The model under review builds one solid part; all positions refer to its coordinate system, in mm. A direction names the side the tool comes from. Give positions to 0.01 mm unless a question says otherwise; leave off trailing zeros. Loops run counter-clockwise (first coordinate to the right, second up) from the corner with the lowest first, then second, coordinate; pieces in that order, holes last. Notation, with made-up numbers: (67, 25) - (95, 25) arc R22 cw to (95, 31) - close; hole circle Ø7 at (18, 55.5). An arc over 180 degrees is marked (long way). Return JSON: item names as keys, results as strings. Group by question number.
```python
from build123d import *

# Parameters (mm, degrees)
SKETCH1_RX          = 20
SKETCH1_RY          = 15
BOSS_EXTRUDE1_DEPTH = 6


with BuildPart() as part:
    # Sketch1 → Boss-Extrude1 (new body)
    with BuildSketch(Plane.XY):
        with BuildLine():
            Line((735.278050496, 436.653824982), (737.672420097, 436.653824982))
            Line((737.672420097, 436.653824982), (737.672420097, 437.878226994))
            Line((737.672420097, 437.878226994), (742.24679609, 437.878226994))
            Line((742.24679609, 437.878226994), (742.24679609, 431.116067))
            Line((742.24679609, 431.116067), (747.348599543, 431.116067))
            Line((747.348599543, 431.116067), (747.348599543, 427.736067))
            Line((747.348599543, 427.736067), (742.114877809, 427.736067))
            ThreePointArc((742.114877809, 427.736067), (721.48448246, 433.262998961), (700.85408711, 427.736067))
            Line((700.85408711, 427.736067), (695.865635692, 427.736067))
            Line((695.865635692, 427.736067), (695.865635692, 431.116067))
            Line((695.865635692, 431.116067), (700.917916144, 431.116067))
            Line((700.917916144, 431.116067), (700.917916144, 437.878226994))
            Line((700.917916144, 437.878226994), (705.492292137, 437.878226994))
            Line((705.492292137, 437.878226994), (705.492292137, 436.653824982))
            Line((705.492292137, 436.653824982), (707.886661739, 436.653824982))
            Line((707.886661739, 436.653824982), (707.886661739, 437.878226994))
            Line((707.886661739, 437.878226994), (709.486661739, 437.878226994))
            Line((709.486661739, 437.878226994), (709.486661739, 440.973907006))
            Line((709.486661739, 440.973907006), (707.886661739, 440.973907006))
            Line((707.886661739, 440.973907006), (707.886661739, 442.198309018))
            Line((707.886661739, 442.198309018), (705.492292137, 442.198309018))
            Line((705.492292137, 442.198309018), (705.492292137, 440.973907006))
            Line((705.492292137, 440.973907006), (700.917916144, 440.973907006))
            Line((700.917916144, 440.973907006), (700.917916144, 459.426067))
            Line((700.917916144, 459.426067), (700.917916144, 477.878226994))
            Line((700.917916144, 477.878226994), (705.492292137, 477.878226994))
            Line((705.492292137, 477.878226994), (705.492292137, 476.653824982))
            Line((705.492292137, 476.653824982), (707.886661739, 476.653824982))
            Line((707.886661739, 476.653824982), (707.886661739, 477.878226994))
            Line((707.886661739, 477.878226994), (709.486661739, 477.878226994))
            Line((709.486661739, 477.878226994), (709.486661739, 480.973907006))
            Line((709.486661739, 480.973907006), (707.886661739, 480.973907006))
            Line((707.886661739, 480.973907006), (707.886661739, 482.198309018))
            Line((707.886661739, 482.198309018), (705.492292137, 482.198309018))
            Line((705.492292137, 482.198309018), (705.492292137, 480.973907006))
            Line((705.492292137, 480.973907006), (700.917916144, 480.973907006))
            Line((700.917916144, 480.973907006), (700.917916144, 487.736067))
            Line((700.917916144, 487.736067), (695.865635692, 487.736067))
            Line((695.865635692, 487.736067), (695.865635692, 491.116067))
            Line((695.865635692, 491.116067), (700.85408711, 491.116067))
            ThreePointArc((700.85408711, 491.116067), (721.48448246, 485.589135038), (742.114877809, 491.116067))
            Line((742.114877809, 491.116067), (747.348599543, 491.116067))
            Line((747.348599543, 491.116067), (747.348599543, 487.736067))
            Line((747.348599543, 487.736067), (742.24679609, 487.736067))
            Line((742.24679609, 487.736067), (742.24679609, 480.973907006))
            Line((742.24679609, 480.973907006), (737.672420097, 480.973907006))
            Line((737.672420097, 480.973907006), (737.672420097, 482.198309018))
            Line((737.672420097, 482.198309018), (735.278050496, 482.198309018))
            Line((735.278050496, 482.198309018), (735.278050496, 480.973907006))
            Line((735.278050496, 480.973907006), (733.799948182, 480.973907006))
            Line((733.799948182, 480.973907006), (733.799948182, 477.878226994))
            Line((733.799948182, 477.878226994), (735.278050496, 477.878226994))
            Line((735.278050496, 477.878226994), (735.278050496, 476.653824982))
            Line((735.278050496, 476.653824982), (737.672420097, 476.653824982))
            Line((737.672420097, 476.653824982), (737.672420097, 477.878226994))
            Line((737.672420097, 477.878226994), (742.24679609, 477.878226994))
            Line((742.24679609, 477.878226994), (742.24679609, 459.426067))
            Line((742.24679609, 459.426067), (742.24679609, 440.973907006))
            Line((742.24679609, 440.973907006), (737.672420097, 440.973907006))
            Line((737.672420097, 440.973907006), (737.672420097, 442.198309018))
            Line((737.672420097, 442.198309018), (735.278050496, 442.198309018))
            Line((735.278050496, 442.198309018), (735.278050496, 440.973907006))
            Line((735.278050496, 440.973907006), (733.799948182, 440.973907006))
            Line((733.799948182, 440.973907006), (733.799948182, 437.878226994))
            Line((733.799948182, 437.878226994), (735.278050496, 437.878226994))
            Line((735.278050496, 437.878226994), (735.278050496, 436.653824982))
        make_face()
        with Locations(Location((721.582356117, 459.426067), (0, 0, 90))):
            Ellipse(SKETCH1_RX, SKETCH1_RY, mode=Mode.SUBTRACT)
    extrude(amount=BOSS_EXTRUDE1_DEPTH)


solid = part.part
```
1) Draft analysis for pull direction Y (two halves, no side actions). For faces 4 (the face through (700.918, 484, 3)), 5 (the face through (721.79, 433.26, 2.96)), 6 (the face through (745, 491.116, 3)), 7 (the face through (735, 437.878, 3)), state which applies: +Y half, -Y half, draft (parallel to the pull), parting line (faces both ways), or undercut.
2) For pin 1 Ø3 at (x, z) = (716.5, 4.5) entering from -Y; pin 2 Ø1 at (y, z) = (481.5, 2.5) entering from +X; pin 3 Ø6 at (x, y) = (741, 441.5) entering from -Z; pin 4 Ø3 at (y, z) = (461, 4.5) entering from -X, all flat-tipped, find the tip position at first contact; note any pin that passes through.
3) We need section A-A, the plane y = 484. Write out the cut boundary in (x, z).
4) To check wall thickness, follow line 1 (Y direction, x = 721.5, z = 4.05); line 2 (X direction, y = 441.5, z = 0.45); line 3 (Y direction, x = 745, z = 4.3). State the ranges of each line that lie inside material, in increasing order.
5) Tool access review of faces 1 (the face through (740, 440.974, 3)), 2 (the face through (707, 482.198, 3)), 3 (the face through (700.918, 434, 3)): name each direction out of +Z, -Z, +X, -X, +Y, -Y from which nothing blocks a thin tool from reaching the whole face with its end or side.
Findings:
{
 "1": {"face 4": "undercut", "face 5": "-Y half", "face 6": "+Y half", "face 7": "undercut"},
 "2": {"pin 1": "stops at y = 432.75", "pin 2": "stops at x = 742.25", "pin 3": "stops at z = 0", "pin 4": "stops at x = 700.92"},
 "3": {"outline": "(700.92, 0) - (742.25, 0) - (742.25, 6) - (700.92, 6) - close"},
 "4": {"line 1": "y = 433.26 to 439.43, 479.43 to 485.59", "line 2": "x = 700.92 to 705.49, 707.89 to 714.93, 728.23 to 735.28, 737.67 to 742.25", "line 3": "y = 427.74 to 431.12, 487.74 to 491.12"},
 "5": {"face 1": "+Z, -Z, +X", "face 2": "+Z, -Z", "face 3": "+Z, -Z, -X"}
}
